```python
from build123d import *

# Parameters (mm, degrees)
SKETCH1_R           = 55
BOSS_EXTRUDE1_DEPTH = 12.7
SKETCH2_R           = 3.2
CUT_EXTRUDE1_DEPTH  = 114.880942125


with BuildPart() as part:
    # Sketch1 → Boss-Extrude1 (new body)
    with BuildSketch(Plane(origin=(0, 0, 0), x_dir=(0, 0, -1), z_dir=(1, 0, 0))):
        Polygon((-62.262586226, 60), (-62.262586226, 42.3), (-74.962586226, 42.3), (-74.962586226, 12.3), (-62.262586226, 12.3), (-62.262586226, -49.4), (-74.962586226, -49.4), (-74.962586226, -79.4), (-62.262586226, -79.4), (-62.262586226, -84.4), (-47.262586226, -84.4), (-47.262586226, -71.7), (-22.262586226, -71.7), (-22.262586226, -84.4), (22.262586226, -84.4), (22.262586226, -71.7), (47.262586226, -71.7), (47.262586226, -84.4), (62.262586226, -84.4), (62.262586226, -66.7), (75.393759552, -66.7), (75.393759552, -36.7), (62.262586226, -36.7), (62.262586226, 12.3), (75.393759552, 12.3), (75.393759552, 42.3), (62.262586226, 42.3), (62.262586226, 60), (47.262586226, 60), (47.262586226, 72.7), (22.262586226, 72.7), (22.262586226, 60), (0, 60), (-22.262586226, 60), (-22.262586226, 72.7), (-47.262586226, 72.7), (-47.262586226, 60), align=None)
        Circle(SKETCH1_R, mode=Mode.SUBTRACT)
    extrude(amount=BOSS_EXTRUDE1_DEPTH)

    # Sketch2 → Cut-Extrude1 (cut, through all)
    with BuildSketch(Plane(origin=(12.7, 0, 0), x_dir=(0, 0, -1), z_dir=(1, 0, 0))):
        with Locations((-62.262586226, 45.5)):
            Circle(SKETCH2_R)
        with Locations((-65.462586226, 12.3)):
            Circle(SKETCH2_R)
        with Locations((-62.262586226, -46.2)):
            Circle(SKETCH2_R)
        with Locations((-65.462586226, -79.4)):
            Circle(SKETCH2_R)
        with Locations((62.262586226, -69.9)):
            Circle(SKETCH2_R)
        with Locations((62.262586226, -33.5)):
            Circle(SKETCH2_R)
        with Locations((65.462586226, 12.3)):
            Circle(SKETCH2_R)
        with Locations((62.262586226, 45.5)):
            Circle(SKETCH2_R)
        with Locations((-50.462586226, 60)):
            Circle(SKETCH2_R)
        with Locations((-19.062586226, 60)):
            Circle(SKETCH2_R)
        with Locations((19.062586226, 60)):
            Circle(SKETCH2_R)
        with Locations((50.462586226, 60)):
            Circle(SKETCH2_R)
        with Locations((-44.062586226, -71.7)):
            Circle(SKETCH2_R)
        with Locations((-25.462586226, -71.7)):
            Circle(SKETCH2_R)
        with Locations((25.462586226, -71.7)):
            Circle(SKETCH2_R)
        with Locations((44.062586226, -71.7)):
            Circle(SKETCH2_R)
    extrude(amount=-CUT_EXTRUDE1_DEPTH, mode=Mode.SUBTRACT)


solid = part.part
```
Here's how the part is built. I have some questions about the finished solid (model axes, mm). A direction names the side the tool comes from. Round coordinates to 2 decimals unless told otherwise and drop trailing zeros. Loops run counter-clockwise (first coordinate to the right, second up) from the corner with the lowest first, then second, coordinate; pieces in that order, holes last. Notation, with made-up numbers: (-12.5, -8) -> (20.5, -8) arc R34 ccw to (20.5, 29) -> close; hole circle Ø11 at (19, 0). An arc over 180 degrees is marked (long way). Answer as CSV lines item,"result".
1. If I drill on L1, parallel to Y at x = 4.5, z = -2; L2, parallel to Z at x = 2.75, y = -76; L3, parallel to Z at x = 11.75, y = 61, over which ranges is the centre line in solid material (lowest first)?
Final values:
L1,"y = -84.4 to -54.96, 54.96 to 60"
L2,"z = -62.26 to -47.26, -22.26 to 22.26, 47.26 to 74.96"
L3,"z = -47.26 to -22.26, 22.26 to 47.26"
2. Thinking about a two-plate mould opening in Z: for faces 5 (the face through (6.439, 45.43, 59.063)), 6 (the face through (6.4, -68.5, 25.4)), 7 (the face through (6.439, -33.43, -59.063)), which applies, released by +Z, released by -Z, zero draft, split by the parting line, or undercut?
Final values:
face 5,"released by +Z"
face 6,"undercut"
face 7,"released by -Z"
3. For pin 1 (4 mm diameter, centred on x = 10, y = -5, fed in from -Z); pin 2 (4 mm diameter, centred on x = 8, y = -5.5, fed in from +Z); pin 3 (3 mm diameter, centred on y = 25, z = -48.5, fed in from +X); pin 4 (4 mm diameter, centred on x = 8, z = -68, fed in from +Y), each with a flat end and sliding along its axis, tell me the tip position at first contact or that it passes through.
Final values:
pin 1,"stops at z = -62.26"
pin 2,"stops at z = 62.26"
pin 3,"stops at x = 12.7"
pin 4,"stops at y = 42.3"
4. If we section it at B-B on y = 35.5: Please give me the cut outline in (x, z), plus the area to 4 significant figures.
Final values:
outline,"(0, -75.39) -> (12.7, -75.39) -> (12.7, -42.01) -> (0, -42.01) -> close; (0, 42.01) -> (12.7, 42.01) -> (12.7, 74.96) -> (0, 74.96) -> close"
area,"842.5 mm^2"
5. If we section it at A-A on y = -7: Please give me the cut outline in (x, z).
Final values:
outline,"(0, -62.26) -> (12.7, -62.26) -> (12.7, -54.55) -> (0, -54.55) -> close; (0, 54.55) -> (12.7, 54.55) -> (12.7, 62.26) -> (0, 62.26) -> close"
6. Which directions (+Z, -Z, +X, -X, +Y, -Y) give clear straight access to the entire face, cutting with the end or side of a thin tool? Please do faces 1 (the face through (6, 54, 62.263)), 2 (the face through (6, -78, -47.263)), 3 (the face through (6, 60, 0)), 4 (the face through (6, 54, -62.263)).
Final values:
face 1,"+Z, +X, -X, +Y"
face 2,"+X, -X, -Y"
face 3,"+X, -X, +Y"
face 4,"-Z, +X, -X, +Y"
